Read the model definition and answer for the solid it produces. Units are mm, in the model's axes. A direction names the side the tool comes from. Round coordinates to 2 decimals unless told otherwise and drop trailing zeros. Order: outer loops, then holes, each group sorted by start corner. A loop starts at its lowest first (then second) coordinate and runs counter-clockwise, first axis right, second up.
from build123d import *

# Parameters (mm, degrees)
F0_W     = 39.6875
F0_H     = 12.7
F4_DEPTH = 12.7
F8_DEPTH = 6.35
F9_W     = 7.9375
F9_H     = 3.175
F11_W    = 7.9375
F11_H    = 3.175


with BuildPart() as f2:
    # F2: sweep along a path in F1
    with BuildLine(Plane.XZ) as f2_path:
        Line((0, 0), (-88.24850028, 0))
        ThreePointArc((-88.24850028, 0), (-112.1747610939, -4.759229181), (-132.4584655909, -18.3123672238))
        Line((-132.4584655909, -18.3123672238), (-188.9358075988, -74.7897092318))
    # F0 (on Right) → F2 (sweep)
    with BuildSketch(Plane.YZ):
        Rectangle(F0_W, F0_H)
    sweep(path=f2_path.line)

    # F3 (on Top) → F4 (cut, symmetric)
    with BuildSketch(Plane.XY):
        with BuildLine():
            Line((-6.35, -2.38125), (0, -2.38125))
            Line((0, -2.38125), (0, 3.96875))
            Line((0, 3.96875), (-6.35, 3.96875))
            ThreePointArc((-6.35, 3.96875), (-16.4659966007, 0.79375), (-6.35, -2.38125))
        make_face()
    extrude(amount=F4_DEPTH, both=True, mode=Mode.SUBTRACT)

    # F7 (on plane+point) → F8 (join, symmetric)
    with BuildSketch(Plane(origin=(-57.0730491835, 0, 57.0730491835), x_dir=(0, -1, 0), z_dir=(-0.7071067812, 0, 0.7071067812))):
        with BuildLine():
            Line((2.38125, -192.8321013228), (2.38125, -186.4821013228))
            Line((2.38125, -186.4821013228), (-3.96875, -186.4821013228))
            Line((-3.96875, -186.4821013228), (-3.96875, -192.8321013228))
            ThreePointArc((-3.96875, -192.8321013228), (-0.79375, -202.9480979235), (2.38125, -192.8321013228))
        make_face()
    extrude(amount=F8_DEPTH, both=True)

    # F10: sweep along a path in F1
    with BuildLine(Plane.XZ) as f10_path:
        Line((0, 0), (-88.24850028, 0))
        ThreePointArc((-88.24850028, 0), (-112.1747610939, -4.759229181), (-132.4584655909, -18.3123672238))
        Line((-132.4584655909, -18.3123672238), (-188.9358075988, -74.7897092318))
    # F9 (on face) → F10 (sweep, cut)
    with BuildSketch(Plane.YZ):
        with Locations((12.4199826866, 4.7625)):
            Rectangle(F9_W, F9_H)
    sweep(path=f10_path.line, mode=Mode.SUBTRACT)

    # F12: sweep along a path in F1
    with BuildLine(Plane.XZ) as f12_path:
        Line((0, 0), (-88.24850028, 0))
        ThreePointArc((-88.24850028, 0), (-112.1747610939, -4.759229181), (-132.4584655909, -18.3123672238))
        Line((-132.4584655909, -18.3123672238), (-188.9358075988, -74.7897092318))
    # F11 (on face) → F12 (sweep, cut)
    with BuildSketch(Plane.YZ):
        with Locations((-11.2668295726, 4.7625)):
            Rectangle(F11_W, F11_H)
    sweep(path=f12_path.line, mode=Mode.SUBTRACT)


solid = f2.part
Q1. A cutting plane is placed at B-B, the plane z = -4. Give the vertices of the cut face in (x, y), plus the area to 3 significant figures.
Outcome:
outline: (-124.56, -19.84) - (0, -19.84) - (0, -2.38) - (-6.35, -2.38) arc R5.56 cw (long way) to (-6.35, 3.97) - (0, 3.97) - (0, 19.84) - (-124.56, 19.84) - (-124.56, 16.39) - (-118.1, 16.39) - (-118.1, 8.45) - (-124.56, 8.45) - (-124.56, -7.3) - (-118.1, -7.3) - (-118.1, -15.24) - (-124.56, -15.24) - close
area: 4,710 mm2
Q2. For faces 1 (the face through (-3, 3.969, 0)), 2 (the face through (-45, 12, 3.175)), 3 (the face through (0, -11, 0)), 4 (the face through (-111.5, 8.451, -0.8)), 5 (the face through (-165.583, 18.14, -42.456)), determine the directions among +Z, -Z, +X, -X, +Y, -Y from which every point of the face is accessible in a straight line to the end or side of a thin tool.
Outcome:
face 1: +Z, -Z, +X
face 2: +Z, +X, -X
face 3: +Z, -Z, +X, +Y, -Y
face 4: +Z, -X
face 5: +Z, -X, +Y, -Y
Q3. For a pull along Y with two mould halves and no side action, classify faces 6 (the face through (-191, 3.969, -77)), 7 (the face through (-45, 1, 6.35)), 8 (the face through (-45, -11, 3.175)) as released by +Y, released by -Y, zero draft, split by the parting line, or undercut.
Outcome:
face 6: released by +Y
face 7: zero draft
face 8: undercut
Q4. Straight lines are drawn through the part: probe 1 along Z at (x, y) = (-18.5, -7); probe 2 along Z at (x, y) = (-35, 14) (3 decimals); probe 3 along X at (y, z) = (-15.5, -77.5). For each, find the intervals that lie inside material, in ascending order.
Outcome:
probe 1: z = -6.35 to 6.35
probe 2: z = -6.35 to 3.175
probe 3: x = -186.23 to -182.67
Q5. Flat-ended cylindrical pins translate along their axes: pin 1 (4 mm diameter, centred on x = -58.5, y = -10.5, fed in from +Z) (3 decimals); pin 2 (3 mm diameter, centred on x = -36, y = -14.5, fed in from -Z); pin 3 (1 mm diameter, centred on x = -126, y = 9.5, fed in from -Z). Find the tip coordinate at first contact, or state that the pin passes through.
Outcome:
pin 1: stops at z = 3.175
pin 2: stops at z = -6.35
pin 3: stops at z = -21.39
Q6. A cutting plane is placed at C-C, the plane x = -54. Give the vertices of the cut face in (y, z) (3 decimals).
Outcome:
outline: (-19.844, -6.35) - (19.844, -6.35) - (19.844, 6.35) - (16.389, 6.35) - (16.389, 3.175) - (8.451, 3.175) - (8.451, 6.35) - (-7.298, 6.35) - (-7.298, 3.175) - (-15.236, 3.175) - (-15.236, 6.35) - (-19.844, 6.35) - close
Q7. A cutting plane is placed at D-D, the plane x = -12.5. Give the vertices of the cut face in (y, z) (3 decimals), plus the area to 3 significant figures.
Outcome:
outline: (-19.844, -6.35) - (-4.53, -6.35) - (-4.53, 6.35) - (-7.298, 6.35) - (-7.298, 3.175) - (-15.236, 3.175) - (-15.236, 6.35) - (-19.844, 6.35) - close; (6.118, -6.35) - (19.844, -6.35) - (19.844, 6.35) - (16.389, 6.35) - (16.389, 3.175) - (8.451, 3.175) - (8.451, 6.35) - (6.118, 6.35) - close
area: 318 mm2
